from build123d import *

# Parameters (mm, degrees)
SKETCH_1_W       = 100
SKETCH_1_H       = 50
EXTRUDE_1_DEPTH  = 10
M10X1_25_1_D     = 8.8
M10X1_25_1_DEPTH = 23.75
M10X1_25_1_TIP   = 2.643786724
FILLET_1_R       = 1
CHAMFER_1_SIZE   = 1
FILLET_2_R       = 1


with BuildPart() as part:
    # 草圖1 → 填料-伸長1 (new body)
    with BuildSketch(Plane(origin=(0, 0, 0), x_dir=(1, 0, 0), z_dir=(0, 1, 0))):
        with Locations((50, 25)):
            Rectangle(SKETCH_1_W, SKETCH_1_H)
    extrude(amount=EXTRUDE_1_DEPTH)

    # M10x1.25 螺紋孔1
    with Locations(Plane(origin=(20, 10, -37.5), x_dir=(0, 0, 1), z_dir=(0, 1, 0))):
        with Locations((0, 0), (25, 0)):
            Hole(M10X1_25_1_D / 2, depth=M10X1_25_1_DEPTH)
            with Locations((0, 0, -(M10X1_25_1_DEPTH + M10X1_25_1_TIP / 2))):  # 118° drill point
                Cone(0, M10X1_25_1_D / 2, M10X1_25_1_TIP, mode=Mode.SUBTRACT)

    # 圓角1
    fillet_1_edges = [part.edges().sort_by_distance(p)[0] for p in [
        (0, 5, -50),
        (100, 5, -50),
        (100, 5, 0),
        (0, 5, 0),
    ]]
    fillet(fillet_1_edges, radius=FILLET_1_R)

    # 導角1
    chamfer_1_edges = [part.edges().sort_by_distance(p)[0] for p in [
        (50, 0, -50),
        (0, 0, -25),
        (100, 0, -25),
        (50, 0, 0),
        (99.707106781, 0, -0.292893219),
        (0.292893219, 0, -0.292893219),
        (0.292893219, 0, -49.707106781),
        (99.707106781, 0, -49.707106781),
    ]]
    chamfer(chamfer_1_edges, length=CHAMFER_1_SIZE)

    # 圓角2
    fillet_2_edges = [part.edges().sort_by_distance(p)[0] for p in [
        (50, 10, -50),
        (100, 10, -25),
        (0, 10, -25),
        (50, 10, 0),
        (99.707106781, 10, -0.292893219),
        (0.292893219, 10, -0.292893219),
        (0.292893219, 10, -49.707106781),
        (99.707106781, 10, -49.707106781),
    ]]
    fillet(fillet_2_edges, radius=FILLET_2_R)


solid = part.part
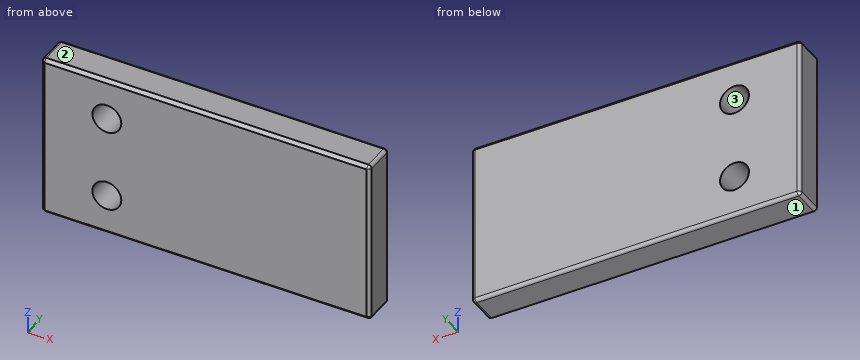
CAD build for the part. Positions are in the model's coordinates, mm. Face numbers are marked on the shaded views. Coordinates: 2 decimals unless noted, no trailing zeros. Order: outer loops, then holes, each group sorted by start corner. A loop starts at its lowest first (then second) coordinate and runs counter-clockwise, first axis right, second up.
Item 1: Band-saw the part on B-B on x = 20. List the corners of the cut face in (y, z).
Check sheet entries:
outline: (0, -49) - (1, -50) - (9, -50) arc R1 ccw to (10, -49) - (10, -41.9) - (0, -41.9) - close; (0, -33.1) - (10, -33.1) - (10, -16.9) - (0, -16.9) - close; (0, -8.1) - (10, -8.1) - (10, -1) arc R1 ccw to (9, 0) - (1, 0) - (0, -1) - close
Item 2: Band-saw the part on C-C on y = 4.5. List the corners of the cut face in (x, z), plus the area to 3 significant figures.
Check sheet entries:
outline: (0, -49) arc R1 ccw to (1, -50) - (99, -50) arc R1 ccw to (100, -49) - (100, -1) arc R1 ccw to (99, 0) - (1, 0) arc R1 ccw to (0, -1) - close; hole circle Ø8.8 at (20, -37.5); hole circle Ø8.8 at (20, -12.5)
area: 4,880 mm2
Item 3: Drill centre lines: L1, parallel to X at y = 6, z = -12.5; L2, parallel to Z at x = 23.5, y = 8; L3, parallel to Z at x = 21, y = 3.75. Where is each one in solid material? Low to high.
Check sheet entries:
L1: x = 0 to 15.6, 24.4 to 100
L2: z = -50 to -40.17, -34.83 to -15.17, -9.83 to 0
L3: z = -50 to -41.78, -33.22 to -16.78, -8.22 to 0
Item 4: Two-plate mould, pull along Z, no slides. Class the marked faces 1, 2 and 3: +Z half, -Z half, draft (parallel to the pull), parting line (faces both ways), or undercut.
Check sheet entries:
face 1: -Z half
face 2: +Z half
face 3: undercut
Item 5: Band-saw the part on A-A on z = -12.5. List the corners of the cut face in (x, y).
Check sheet entries:
outline: (0, 1) - (1, 0) - (15.6, 0) - (15.6, 10) - (1, 10) arc R1 ccw to (0, 9) - close; (24.4, 0) - (99, 0) - (100, 1) - (100, 9) arc R1 ccw to (99, 10) - (24.4, 10) - close
